Part print with two shaded views. Sizes in mm from the minimum x, y, z corner. Coordinates: 2 decimals unless noted, no trailing zeros. Loops run counter-clockwise (first coordinate to the right, second up) from the corner with the lowest first, then second, coordinate; pieces in that order, holes last. Notation, with made-up numbers: (79, -40) -> (108, -40) arc R16 ccw to (108, -9) -> close; hole circle Ø10 at (53.25, 26). An arc over 180 degrees is marked (long way). Write each question's results on one line, items separated by ' | '.
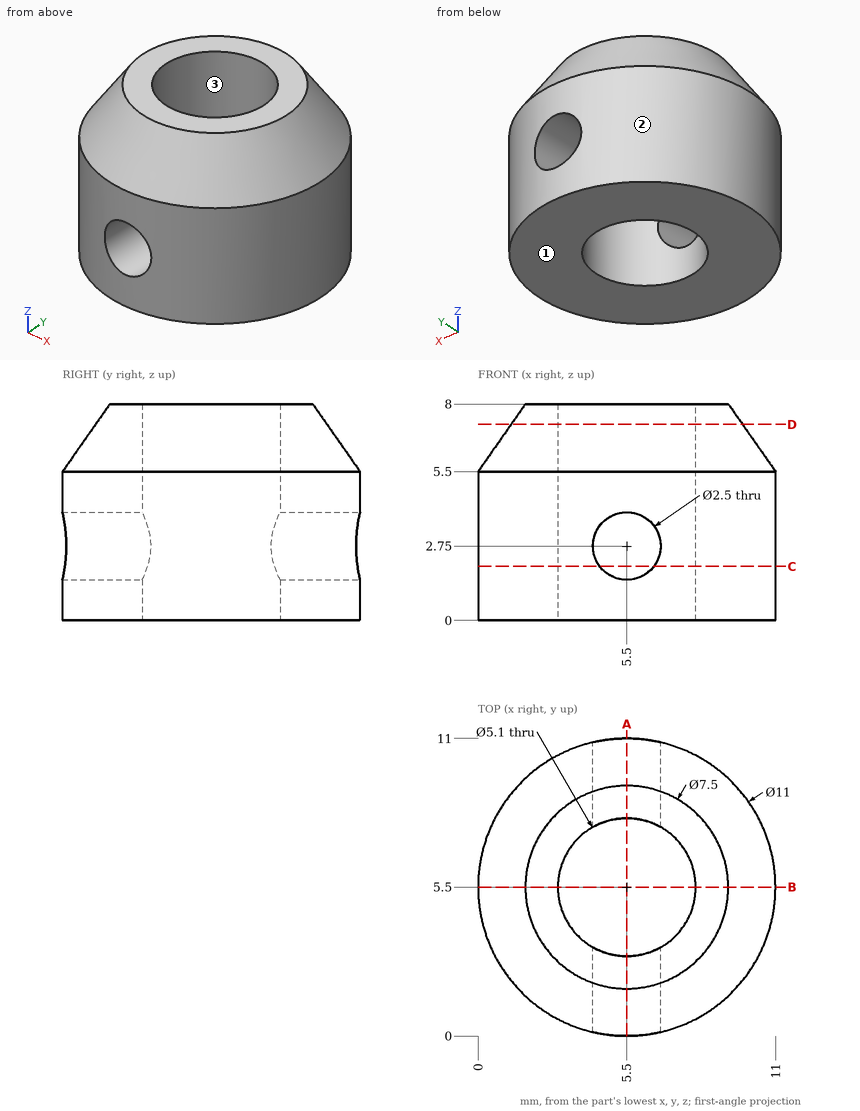
Q1. Drop flat-ended pins along their axis: pin 1 (1.5 mm diameter, centred on y = 4, z = 6.5, fed in from -X); pin 2 (1 mm diameter, centred on y = 9, z = 6.5, fed in from +X); pin 3 (4 mm diameter, centred on x = 8, z = 2, fed in from -Y). Give the stop position or say it passes through.
Results are:
pin 1: x = 0.35 | pin 2: x = 9.45 | pin 3: y = 0.03
Q2. Pull direction Y, two halves, no side cores. Call the marked faces 1, 2 and 3: +Y half, -Y half, draft (parallel to the pull), parting line (faces both ways), or undercut.
Results are:
face 1: draft | face 2: parting line | face 3: undercut
Q3. Wall check: L1, parallel to Y at x = 3.75, z = 0.5; L2, parallel to Y at x = 3.5, z = 7.25; L3, parallel to X at y = 4, z = 5.75. Give the ranges that are in metal, low to high. Write a range as from..to.
Results are:
L1: 0.29..3.65, 7.35..10.71 | L2: 1.72..3.92, 7.08..9.28 | L3: 0.39..3.44, 7.56..10.61
Q4. Cut at A-A on x = 5.5. Write the cut outline in (y, z).
Results are:
outline: (0, 0) -> (2.95, 0) -> (2.95, 1.5) -> (0, 1.5) -> close; (0, 4) -> (2.95, 4) -> (2.95, 8) -> (1.75, 8) -> (0, 5.5) -> close; (8.05, 0) -> (11, 0) -> (11, 1.5) -> (8.05, 1.5) -> close; (8.05, 4) -> (11, 4) -> (11, 5.5) -> (9.25, 8) -> (8.05, 8) -> close
Q5. Cut at B-B on y = 5.5. Write the cut outline in (x, z), and give its area (3 significant figures).
Results are:
outline: (0, 0) -> (2.95, 0) -> (2.95, 8) -> (1.75, 8) -> (0, 5.5) -> close; (8.05, 0) -> (11, 0) -> (11, 5.5) -> (9.25, 8) -> (8.05, 8) -> close | area: 42.8 mm^2
Q6. Cut at D-D on z = 7.25. Write the cut outline in (x, y) (3 decimals).
Results are:
outline: circle Ø8.55 at (5.5, 5.5); hole circle Ø5.1 at (5.5, 5.5)
Q7. Cut at C-C on z = 2. Write the cut outline in (x, y), and give its area (3 significant figures).
Results are:
outline: (4.5, 0.09) -> (4.5, 3.15) arc R2.55 cw to (4.5, 7.85) -> (4.5, 10.91) arc R5.5 ccw to start; (6.5, 0.09) arc R5.5 ccw to (6.5, 10.91) -> (6.5, 7.85) arc R2.55 cw to (6.5, 3.15) -> close | area: 62.7 mm^2
